Here's how the part is built. I have some questions about the finished solid (model axes, mm). A direction names the side the tool comes from. Coordinates: 2 decimals unless noted, no trailing zeros. Write each loop counter-clockwise with the first axis right and the second up, starting at its lowest first coordinate (ties: lowest second). Pieces come first, ordered by that corner, then holes. Notation, with made-up numbers: (-9.75, -29) - (45.25, -29) arc R20 ccw to (45.25, -25) - close; hole circle Ø1 at (-12.5, -3). An arc over 180 degrees is marked (long way). Answer in a Markdown table with one row per item. Add a question column.
Item 1: Which directions (+Z, -Z, +X, -X, +Y, -Y) give clear straight access to the entire face, cutting with the end or side of a thin tool? Please do faces 4 (the face through (9.16, -6.19, 1.48)), 5 (the face through (52, 0.5, 1)).
Item 2: We'd pull the mould along Y, two halves only. Please class faces 1 (the face through (19.6, 46.5, 1.5)), 2 (the face through (46, 31, 0)), 3 (the face through (-8.28, -5.87, 1.48)): +Y half, -Y half, draft (parallel to the pull), parting line (faces both ways), or undercut.
Item 3: If I drill on probe 1 along Y at (x, z) = (-8, 0.8); probe 2 along Y at (x, z) = (57, 2.5); probe 3 along X at (y, z) = (7, 1.8), over which ranges is the centre line in solid material (lowest first)? Write a range as from..to.
Item 4: Imagine slicing it at D-D (x = 47). Please give me the cut outline in (y, z).
Item 5: Imagine slicing it at C-C (z = 2.1). Please give me the cut outline in (x, y), plus the area to 3 significant figures.
Item 6: Imagine slicing it at A-A (y = -8). Please give me the cut outline in (x, z).
Item 7: I'm going to push flat-ended pins straight in: pin 1 (5 mm diameter, centred on x = 8, y = -8, fed in from -Z); pin 2 (4 mm diameter, centred on x = -8, y = -8, fed in from +Z). Where does each tip first touch, or does it pass through?
Item 8: Imagine slicing it at B-B (x = 8). Please give me the cut outline in (y, z).
from build123d import *

# Parameters (mm, degrees)
SKETCH_R   = 2.15
SKETCH_R_2 = 5
PAD_DEPTH  = 3


with BuildPart() as part:
    # Sketch → Pad (new body)
    with BuildSketch(Plane.XY):
        with BuildLine():
            Line((36.7, 0.5), (84.5, 0.5))
            ThreePointArc((84.5, 0.5), (85.914214, 1.085786), (86.5, 2.5))
            Line((86.5, 2.5), (86.5, 74.7))
            ThreePointArc((86.5, 74.7), (85.914214, 76.114214), (84.5, 76.7))
            Line((84.5, 76.7), (37.865935, 76.7))
            ThreePointArc((37.865935, 76.7), (36.858665, 76.427833), (36.12554, 75.685406))
            Line((3.48079, 18.029189), (36.12554, 75.685406))
            ThreePointArc((0, 16), (2.014541, 16.544335), (3.48079, 18.029189))
            ThreePointArc((0, 16), (-12.263768, -10.276186), (15.753095, -2.8))
            ThreePointArc((19.691369, 0.5), (17.122322, -0.434058), (15.753095, -2.8))
            Line((36.7, 0.5), (19.691369, 0.5))
        make_face()
        with Locations((-8, 8)):
            Circle(SKETCH_R, mode=Mode.SUBTRACT)
        with Locations((8, 8)):
            Circle(SKETCH_R, mode=Mode.SUBTRACT)
        with Locations((-8, -8)):
            Circle(SKETCH_R, mode=Mode.SUBTRACT)
        with Locations((8, -8)):
            Circle(SKETCH_R, mode=Mode.SUBTRACT)
        Circle(SKETCH_R_2, mode=Mode.SUBTRACT)
    extrude(amount=PAD_DEPTH)


solid = part.part
Here are the results:
| question | item | result |
|---|---|---|
| 1 | face 4 | +Z, -Z |
| 1 | face 5 | +Z, -Z, +X, -Y |
| 2 | face 1 | +Y half |
| 2 | face 2 | draft |
| 2 | face 3 | undercut |
| 3 | probe 1 | y = -13.86..-10.15, -5.85..5.85, 10.15..13.86 |
| 3 | probe 2 | y = 0.5..76.7 |
| 3 | probe 3 | x = -14.39..-9.9, -6.1..6.1, 9.9..86.5 |
| 4 | outline | (0.5, 0) - (76.7, 0) - (76.7, 3) - (0.5, 3) - close |
| 5 | outline | (0, 16) arc R16 ccw (long way) to (15.75, -2.8) arc R4 cw to (19.69, 0.5) - (84.5, 0.5) arc R2 ccw to (86.5, 2.5) - (86.5, 74.7) arc R2 ccw to (84.5, 76.7) - (37.87, 76.7) arc R2 ccw to (36.13, 75.69) - (3.48, 18.03) arc R4 cw to start; hole circle Ø4.3 at (-8, -8); hole circle Ø4.3 at (-8, 8); hole circle Ø10 at (0, 0); hole circle Ø4.3 at (8, -8); hole circle Ø4.3 at (8, 8) |
| 5 | area | 5,880 mm2 |
| 6 | outline | (-13.86, 0) - (-10.15, 0) - (-10.15, 3) - (-13.86, 3) - close; (-5.85, 0) - (5.85, 0) - (5.85, 3) - (-5.85, 3) - close; (10.15, 0) - (13.86, 0) - (13.86, 3) - (10.15, 3) - close |
| 7 | pin 1 | stops at z = 0 |
| 7 | pin 2 | passes through |
| 8 | outline | (-13.86, 0) - (-10.15, 0) - (-10.15, 3) - (-13.86, 3) - close; (-5.85, 0) - (5.85, 0) - (5.85, 3) - (-5.85, 3) - close; (10.15, 0) - (26.01, 0) - (26.01, 3) - (10.15, 3) - close |
